```python
from build123d import *

# Parameters (mm, degrees)
BOSS_EXTRUDE2_DEPTH                            = 63.5
SHELL1_T                                       = -2.54
BOSS_EXTRUDE4_DEPTH                            = 25.4
FILLET1_R                                      = 2.54
CSK_FOR_6_FLAT_HEAD_MACHINE_SCREW2_D           = 3.7973
CSK_FOR_6_FLAT_HEAD_MACHINE_SCREW2_DEPTH       = 4.7625
CSK_FOR_6_FLAT_HEAD_MACHINE_SCREW2_CSINK_D     = 7.0866
CSK_FOR_6_FLAT_HEAD_MACHINE_SCREW2_CSINK_ANGLE = 82
CSK_FOR_6_FLAT_HEAD_MACHINE_SCREW1_D           = 3.7973
CSK_FOR_6_FLAT_HEAD_MACHINE_SCREW1_CSINK_D     = 7.0866
CSK_FOR_6_FLAT_HEAD_MACHINE_SCREW1_CSINK_ANGLE = 82
CUT_EXTRUDE1_REACH                             = 110.657
SKETCH10_R                                     = 3.5
BOSS_EXTRUDE6_START                            = 3.175
BOSS_EXTRUDE6_DEPTH                            = 3.175
SKETCH15_R                                     = 6
CUT_EXTRUDE2_DEPTH                             = 38.735


with BuildPart() as part:
    # Sketch4 → Boss-Extrude2 (new body)
    with BuildSketch(Plane(origin=(0, 0, 0), x_dir=(0, 0, -1), z_dir=(1, 0, 0))):
        Polygon((0, 50.8), (-38.100141797, 0), (0, 0), align=None)
    extrude(amount=BOSS_EXTRUDE2_DEPTH)

    # Shell1
    shell1_openings = [part.faces().sort_by_distance(p)[0] for p in [
        (31.75, 0, 19.050070899),
    ]]
    offset(amount=SHELL1_T, openings=shell1_openings, kind=Kind.INTERSECTION)

    # Sketch5 → Boss-Extrude4 (add)
    with BuildSketch(Plane(origin=(0, 18.28808712, 24.38402541), x_dir=(1, 0, 0), z_dir=(0, 0.6000014291326663, 0.7999989281485057))):
        Polygon((12.7, -22.860139528), (12.7, -7.620139528), (15.875, -7.620139528), (15.875, -5.080139528), (0, 40.63994555), (0, 17.779903011), (7.9375, -5.080139528), (7.9375, -22.860139528), align=None)
        Polygon((55.5625, -5.080139528), (55.5625, -22.860139528), (50.8, -22.860139528), (50.8, -7.620139528), (47.625, -7.620139528), (47.625, -5.080139528), (63.5, 40.63994555), (63.5, 17.779903011), align=None)
    extrude(amount=BOSS_EXTRUDE4_DEPTH)

    # Fillet1
    fillet1_edges = [part.edges().sort_by_distance(p)[0] for p in [
        (15.875, 21.843999092, 37.592102775),
        (47.625, 21.843999092, 37.592102775),
    ]]
    fillet(fillet1_edges, radius=FILLET1_R)

    # CSK for #6 Flat Head Machine Screw2
    with Locations(Plane.ZY.offset(-7.9375)):
        with Locations((43.688117295, 13.716009982)):
            CounterSinkHole(CSK_FOR_6_FLAT_HEAD_MACHINE_SCREW2_D / 2, CSK_FOR_6_FLAT_HEAD_MACHINE_SCREW2_CSINK_D / 2, depth=CSK_FOR_6_FLAT_HEAD_MACHINE_SCREW2_DEPTH, counter_sink_angle=CSK_FOR_6_FLAT_HEAD_MACHINE_SCREW2_CSINK_ANGLE)

    # CSK for #6 Flat Head Machine Screw1 (through all)
    with Locations(Plane(origin=(55.5625, 0, 0), x_dir=(0, 0, -1), z_dir=(1, 0, 0))):
        with Locations((-43.688117295, 13.716009982)):
            CounterSinkHole(CSK_FOR_6_FLAT_HEAD_MACHINE_SCREW1_D / 2, CSK_FOR_6_FLAT_HEAD_MACHINE_SCREW1_CSINK_D / 2, counter_sink_angle=CSK_FOR_6_FLAT_HEAD_MACHINE_SCREW1_CSINK_ANGLE)

    # Sketch10 → Cut-Extrude1 (cut, up to next)
    with BuildSketch(Plane(origin=(0, 0, 0), x_dir=(-1, 0, 0), z_dir=(0, 0, -1)), mode=Mode.PRIVATE) as cut_extrude1_sk1:
        with Locations((-31.75, 35.8)):
            Circle(SKETCH10_R)
    cut_extrude1_tool1 = extrude(cut_extrude1_sk1.sketch, amount=-CUT_EXTRUDE1_REACH, mode=Mode.PRIVATE) & part.part
    add(cut_extrude1_tool1.solids().sort_by_distance((31.75, 35.8, 0))[0], mode=Mode.SUBTRACT)

    # Sketch11 → Boss-Extrude6 (add)
    with BuildSketch(Plane(origin=(0, 18.28808712, 24.38402541), x_dir=(1, 0, 0), z_dir=(0, 0.6000014291326664, 0.7999989281485057)).offset(BOSS_EXTRUDE6_START)):
        with BuildLine():
            Line((1.763885607, 35.55994555), (61.736114393, 35.55994555))
            Line((61.736114393, 35.55994555), (47.765528412, -4.675416947))
            ThreePointArc((47.765528412, -4.675416947), (47.660378488, -5.086106873), (47.625, -5.508565254))
            Line((47.625, -5.508565254), (47.625, -7.620139528))
            Line((47.625, -7.620139528), (15.875, -7.620139528))
            Line((15.875, -7.620139528), (15.875, -5.508565254))
            ThreePointArc((15.875, -5.508565254), (15.839621512, -5.086106873), (15.734471588, -4.675416947))
            Line((15.734471588, -4.675416947), (1.763885607, 35.55994555))
        make_face()
    extrude(amount=-BOSS_EXTRUDE6_DEPTH)

    # Sketch14 → Loft2 section 0
    with BuildSketch(Plane(origin=(12.592837865, 3.497999322, -2.623509255), x_dir=(-0.16778323619732566, -0.12899238858965661, -0.9773483254894785), z_dir=(0.9446738533698645, 0.2624085638294688, -0.19680715532796914))):
        with BuildLine():
            Line((-6.55281334, 48.579854588), (-12.031696709, 45.583164002))
            Line((-12.031696709, 45.583164002), (-9.303504202, 43.959097917))
            Line((-9.303504202, 43.959097917), (-6.55281334, 48.579854588))
        make_face()
    # Sketch12 → Loft2 section 1
    with BuildSketch(Plane(origin=(44.075113902, -12.243048009, 9.182320181), x_dir=(-0.16312891841524135, 0.1446897924855975, 0.9759374057423705), z_dir=(-0.9446738533698645, 0.26240856382946876, -0.19680715532796894))):
        with BuildLine():
            Line((2.42045406, 63.449507231), (-3.008444861, 66.535827684))
            Line((-3.008444861, 66.535827684), (-0.334058341, 61.870492844))
            Line((-0.334058341, 61.870492844), (2.42045406, 63.449507231))
        make_face()
    loft()

    # Sketch15 → Cut-Extrude2 (cut)
    with BuildSketch(Plane.XY.offset(2.54)):
        with Locations(Location((31.75, 35.8, 0), (0, 0, 90))):
            Circle(SKETCH15_R)
    extrude(amount=CUT_EXTRUDE2_DEPTH, mode=Mode.SUBTRACT)


solid = part.part
```
Geometry: final body of the model. Coordinates: model frame, mm. A direction names the side the tool comes from. Coordinates: 2 decimals unless noted, no trailing zeros. Order: outer loops, then holes, each group sorted by start corner. A loop starts at its lowest first (then second) coordinate and runs counter-clockwise, first axis right, second up. Notation, with made-up numbers: (73, -6.5) -> (106, -6.5) arc R27 cw to (106, 24.5) -> close; hole circle Ø10 at (20, 9.25). An arc over 180 degrees is marked (long way). Answer in a Markdown table with one row per item.
Item 1: Access query for faces 1 (the flat face through (31.483, 6.181, 33.464)), 2 (the flat face through (8, 40, 24)), 3 (the flat face through (7.938, 18, 44)). Directions: +Z, -Z, +X, -X, +Y, -Y. A direction counts if a zero-diameter tool reaches every point of the face in a straight line with its end or side. Return the directions, or none.
Return value:
| item | result |
|---|---|
| face 1 | +Z |
| face 2 | +Y |
| face 3 | +Z, -X |
Item 2: Ray query, L1, parallel to X at y = 23, z = 50.5; L2, parallel to X at y = 18, z = 10; L3, parallel to Y at x = 31.75, z = 0.9. Return the intervals inside material, ascending.
Return value:
| item | result |
|---|---|
| L1 | x = 7.94 to 12.7, 50.8 to 55.56 |
| L2 | x = 0 to 2.54, 60.96 to 63.5 |
| L3 | y = 0 to 32.3, 39.3 to 50.45 |
Item 3: Draft query along X for faces 4 (the flat face through (30.43, 13.64, 30.89)), 5 (the flat face through (55.6, 38.88, 40.69)), 6 (the flat face through (50.8, 12, 41)), 7 (the flat face through (3.913, 31.009, 30.496)). Return one class per face: released by +X, released by -X, zero draft, split by the parting line, or undercut.
Return value:
| item | result |
|---|---|
| face 4 | undercut |
| face 5 | zero draft |
| face 6 | undercut |
| face 7 | released by -X |
Item 4: Contact query for flat-ended pins moving along their axis: P1, Ø5, axis at y = 13.72, z = 43.69, coming from the +X side; P2, Ø6, axis at x = 32.5, y = 47.5, coming from the +Z side; P3, Ø9, axis at y = 12, z = 46.5, coming from the +X side; P4, Ø5, axis at x = 27.5, z = 42, coming from the -Y side. Output: stop coordinate, or through.
Return value:
| item | result |
|---|---|
| P1 | stops at x = 54.37 |
| P2 | stops at z = 8.69 |
| P3 | stops at x = 55.56 |
| P4 | passes through |
Item 5: Section C-C on y = 54. Output: boundary loops of the cut face in (x, z), plus the area to 3 significant figures.
Return value:
| item | result |
|---|---|
| outline | (0, 4.27) -> (5.23, 29.35) -> (0, 29.35) -> close; (58.27, 29.35) -> (63.5, 4.27) -> (63.5, 29.35) -> close |
| area | 131 mm² |
Item 6: Section B-B on x = 31.75. State how many separate pieces and enclosed holes the cut face has, plus the area to 3 significant figures.
Return value:
| item | result |
|---|---|
| separate pieces | 3 |
| enclosed holes | 0 |
| area | 310 mm² |
